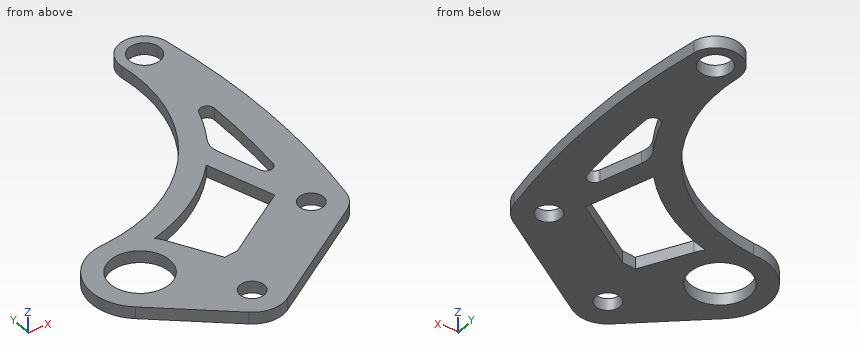
```python
from build123d import *

# Parameters (mm, degrees)
SKETCH2_R           = 7.9375
SKETCH2_R_2         = 3.2639
SKETCH2_R_3         = 4.191
BOSS_EXTRUDE1_DEPTH = 3.175
FILLET3_R           = 1.905
FILLET4_R           = 6.35


with BuildPart() as part:
    # Sketch2 → Boss-Extrude1 (new body)
    with BuildSketch(Plane.XY):
        with BuildLine():
            ThreePointArc((53.924522294, -1.518710351), (57.106411985, 32.846575285), (54.035830718, 67.22198524))
            ThreePointArc((54.035830718, 67.22198524), (46.333024889, 72.662028043), (40.750647472, 65.061742146))
            ThreePointArc((40.750647472, 65.061742146), (31.550758366, 30.452598432), (0.230104832, 13.090356345))
            Line((0.230104832, 13.090356345), (0.171615761, 13.016368706))
            ThreePointArc((0.171615761, 13.016368706), (-12.221668504, 4.481754704), (-8.283857999, -10.041563768))
            Line((-8.283857999, -10.041563768), (10.974906006, -25.929215326))
            ThreePointArc((10.974906006, -25.929215326), (15.847415014, -27.825253688), (20.891605497, -26.449590983))
            Line((20.891605497, -26.449590983), (50.326948559, -6.956773116))
            ThreePointArc((50.326948559, -6.956773116), (52.678920751, -4.603703856), (53.924522294, -1.518710351))
        make_face()
        Circle(SKETCH2_R, mode=Mode.SUBTRACT)
        with Locations((16.284656938, -19.492817867)):
            Circle(SKETCH2_R_2, mode=Mode.SUBTRACT)
        with Locations((45.72, 0)):
            Circle(SKETCH2_R_2, mode=Mode.SUBTRACT)
        with BuildLine():
            Line((40.587817362, 6.608950017), (21.967466437, -5.721910488))
            Line((21.967466437, -5.721910488), (18.339656124, -6.094706177))
            Line((18.339656124, -6.094706177), (11.355144297, 6.365218318))
            ThreePointArc((11.355144297, 6.365218318), (10.656204093, 7.476671758), (9.848859751, 8.512066016))
            ThreePointArc((9.848859751, 8.512066016), (23.445327069, 14.632175726), (34.749899024, 24.354640398))
            Line((34.749899024, 24.354640398), (40.587817362, 6.608950017))
        make_face(mode=Mode.SUBTRACT)
        with BuildLine():
            ThreePointArc((47.523781163, 56.501393309), (48.257752726, 32.370804269), (45.933946154, 8.34115665))
            Line((45.933946154, 8.34115665), (38.882442516, 29.775817606))
            ThreePointArc((38.882442516, 29.775817606), (45.039190515, 42.544935267), (47.523781163, 56.501393309))
        make_face(mode=Mode.SUBTRACT)
        with Locations((47.413333333, 66.018287029)):
            Circle(SKETCH2_R_3, mode=Mode.SUBTRACT)
    extrude(amount=BOSS_EXTRUDE1_DEPTH)

    # Fillet3
    fillet3_edges = [part.edges().sort_by_distance(p)[0] for p in [
        (47.523781163, 56.501393309, 1.5875),
        (45.933946154, 8.34115665, 1.5875),
    ]]
    fillet(fillet3_edges, radius=FILLET3_R)

    # Fillet4
    fillet4_edges = [part.edges().sort_by_distance(p)[0] for p in [
        (38.882442516, 29.775817606, 1.5875),
    ]]
    fillet(fillet4_edges, radius=FILLET4_R)


solid = part.part
```
Work out the finished part from the listing and answer in its coordinate system (mm). Give positions to 0.01 mm unless a question says otherwise; leave off trailing zeros. Loops run counter-clockwise (first coordinate to the right, second up) from the corner with the lowest first, then second, coordinate; pieces in that order, holes last. Notation, with made-up numbers: (-18.75, 11.25) -> (-5.75, 11.25) arc R23 ccw to (-5.75, 49.25) -> close; hole circle Ø10 at (68, 21). An arc over 180 degrees is marked (long way). Use CSV: the item, a comma, the result in double quotes.
1. The part is cut by section D-D (y = 1.5). Write down the section's boundary in (x, z) (3 decimals).
Found:
outline,"(-12.931, 0) -> (-7.794, 0) -> (-7.794, 3.175) -> (-12.931, 3.175) -> close; (7.794, 0) -> (14.082, 0) -> (14.082, 3.175) -> (7.794, 3.175) -> close; (32.873, 0) -> (42.821, 0) -> (42.821, 3.175) -> (32.873, 3.175) -> close; (48.619, 0) -> (54.458, 0) -> (54.458, 3.175) -> (48.619, 3.175) -> close"
2. Straight lines are drawn through the part: line 1 (X direction, y = 24, z = 0.6); line 2 (Y direction, x = 45.72, z = 2.25); line 3 (Y direction, x = -1, z = 2.7). For each, find the intervals that lie inside material, in ascending order.
Found:
line 1,"25.42 to 34.44, 34.87 to 40.78, 47.8 to 56.89"
line 2,"-10.01 to -3.26, 3.26 to 14.91, 42.51 to 62.18, 69.85 to 72.53"
line 3,"-16.05 to -7.87, 7.87 to 12.98"
3. The part is cut by section B-B (x = 4). Write down the section's boundary in (y, z) (3 decimals).
Found:
outline,"(-20.175, 0) -> (-6.856, 0) -> (-6.856, 3.175) -> (-20.175, 3.175) -> close; (6.856, 0) -> (13.643, 0) -> (13.643, 3.175) -> (6.856, 3.175) -> close"
4. The part is cut by section A-A (y = 31). Write down the section's boundary in (x, z) (3 decimals), then the cut area to 3 significant figures.
Found:
outline,"(31.971, 0) -> (39.839, 0) -> (39.839, 3.175) -> (31.971, 3.175) -> close; (48.208, 0) -> (57.094, 0) -> (57.094, 3.175) -> (48.208, 3.175) -> close"
area,"53.2 mm^2"
5. The part is cut by section C-C (y = 18). Write down the section's boundary in (x, z) (3 decimals), then the cut area to 3 significant figures.
Found:
outline,"(16.586, 0) -> (28.141, 0) -> (28.141, 3.175) -> (16.586, 3.175) -> close; (36.84, 0) -> (42.756, 0) -> (42.756, 3.175) -> (36.84, 3.175) -> close; (47.238, 0) -> (56.503, 0) -> (56.503, 3.175) -> (47.238, 3.175) -> close"
area,"84.9 mm^2"
